Design review of the part built by this model. Coordinates are the model's own, in mm. Give positions to 0.01 mm unless a question says otherwise; leave off trailing zeros. Loops run counter-clockwise (first coordinate to the right, second up) from the corner with the lowest first, then second, coordinate; pieces in that order, holes last. Notation, with made-up numbers: M -9.75,75.25 L 16.25,75.25 A26 cw 16.25,109.25 Z; hole C 89,57.25 d8. An arc over 180 degrees is marked long. Use CSV: the item, a comma, the result in double quotes.
from build123d import *

# Parameters (mm, degrees)
SKETCH1_R      = 6.6929
SKETCH1_R_2    = 2.6289
EXTRUDE1_DEPTH = 0.635
EXTRUDE2_START = -0.635
EXTRUDE2_DEPTH = 0.635
SKETCH5_W      = 3.145443006
SKETCH5_H      = 4.115631968
EXTRUDE3_DEPTH = 0.635


# Read off the part's stored shape, not the designer's step: Extrude2
with BuildPart() as part:
    # Sketch1 → Extrude1 (new body)
    with BuildSketch(Plane.XY):
        Circle(SKETCH1_R)
        Circle(SKETCH1_R_2, mode=Mode.SUBTRACT)
    extrude(amount=EXTRUDE1_DEPTH)

    # Extrude2 outline → Extrude2 (cut)
    with BuildSketch(Plane.XY.offset(0.635).offset(EXTRUDE2_START)):
        with BuildLine():
            Line((4.778033454, -4.686715984), (-4.778033454, -4.686715984))
            ThreePointArc((-4.778033454, -4.686715984), (0, -6.6929), (4.778033454, -4.686715984))
        make_face()
    extrude(amount=EXTRUDE2_DEPTH, mode=Mode.SUBTRACT)

    # Sketch5 → Extrude3 (cut)
    with BuildSketch(Plane.XY.offset(0.635)):
        with Locations((0, -2.6289)):
            Rectangle(SKETCH5_W, SKETCH5_H)
    extrude(amount=-EXTRUDE3_DEPTH, mode=Mode.SUBTRACT)


solid = part.part
(1) Clearance check with a flat-ended pin moving along its axis: P1, Ø2, axis at x = 0.5, y = -2, coming from the -Z side. State where the tip first meets the part, or that it passes through.
A:
P1,"through"
(2) We need section D-D on x = 0. State the section outline as (y, z) points (3 decimals), then the cut area to 3 significant figures.
A:
outline,"M 2.629,0 L 6.693,0 L 6.693,0.635 L 2.629,0.635 Z"
area,"2.58 mm²"
(3) We need section A-A on y = 0. State the section outline as (x, z) points (3 decimals), then the cut area to 3 significant figures.
A:
outline,"M -6.693,0 L -2.629,0 L -2.629,0.635 L -6.693,0.635 Z; M 2.629,0 L 6.693,0 L 6.693,0.635 L 2.629,0.635 Z"
area,"5.16 mm²"
(4) We need section C-C on z = 0.25. State the section outline as (x, y) points, then the cut area to 3 significant figures.
A:
outline,"M -4.78,-4.69 L -1.57,-4.69 L -1.57,-2.11 A2.63 cw long 1.57,-2.11 L 1.57,-4.69 L 4.78,-4.69 A6.69 ccw long Z"
area,"98.8 mm²"
(5) We need section B-B on x = 2.25. State the section outline as (y, z) points (3 decimals).
A:
outline,"M -4.687,0 L -1.36,0 L -1.36,0.635 L -4.687,0.635 Z; M 1.36,0 L 6.303,0 L 6.303,0.635 L 1.36,0.635 Z"
(6) The part is to be moulded in two halves that separate along Y. For faces 1 (the cylindrical face through (0.22, 6.69, 0.31)), 2 (the flat face through (-2, 2, 0.635)), 3 (the cylindrical face through (0.092, 2.627, 0.313)), say which applies: released by +Y, released by -Y, zero draft, split by the parting line, or undercut.
A:
face 1,"split by the parting line"
face 2,"zero draft"
face 3,"undercut"
(7) Wall thickness on line 1 along X through (y, z) = (0, 0.45); line 2 along X through (y, z) = (-2.25, 0.2); line 3 along Y through (x, z) = (0, 0.35): over which ranges is each line inside the solid? List them lowest first. Write a range as [from, to].
A:
line 1,"[-6.69, -2.63], [2.63, 6.69]"
line 2,"[-6.3, -1.57], [1.57, 6.3]"
line 3,"[2.63, 6.69]"
